The listing builds one solid part. Answer for the finished solid, in the listing's coordinates (mm). Face numbers are marked on the shaded views. A direction names the side the tool comes from. Round coordinates to 2 decimals unless told otherwise and drop trailing zeros. Loops run counter-clockwise (first coordinate to the right, second up) from the corner with the lowest first, then second, coordinate; pieces in that order, holes last. Notation, with made-up numbers: (55, 18) -> (84, 18) arc R28 cw to (84, 52) -> close; hole circle Ø3 at (41, 65.25). An arc over 180 degrees is marked (long way). Use a Markdown table: item, result. Add a question column.
Q1. Which of the six approach directions +Z, -Z, +X, -X, +Y, -Y give full straight-line access (tool end or side, diameter ignored) to the marked faces 1, 2 and 3?
Q2. Section A-A on x = -14.5 is taken. Give the vertices of the cut face in (y, z), then the cut area to 4 significant figures.
Q3. Given pin 1 Ø1.1 at (x, y) = (-13, 10.5) entering from +Z; pin 2 Ø14.5 at (x, y) = (-2, 2.5) entering from +Z; pin 3 Ø1.6 at (y, z) = (4, 1) entering from +X (3 decimals); pin 4 Ø1.1 at (y, z) = (5.5, 1) entering from -X (3 decimals), each flat-ended and moving along its own axis, determine where each tip first touches the part or whether it passes through.
Q4. Section B-B on x = 11.5 is taken. Give the vertices of the cut face in (y, z).
Q5. Consider line 1 (Y direction, x = 7, z = 0.6); line 2 (Y direction, x = 8.5, z = 2.85); line 3 (Y direction, x = 10, z = 0.5). Determine where each line is inside the solid, lowest interval first.
Q6. Section C-C on y = 5.5 is taken. Give the vertices of the cut face in (x, z) (3 decimals).
Q7. Section D-D on x = 0 is taken. Give the vertices of the cut face in (y, z).
from build123d import *

# Parameters (mm, degrees)
SKETCH_1_W            = 26.05
SKETCH_1_H            = 25
EXTRUDE_1_DEPTH       = 1.5
SKETCH_3_W            = 5.4
SKETCH_3_H            = 11.2
CUT_EXTRUDE_1_DEPTH   = 19.114928236
SKETCH_4_W            = 26.05
SKETCH_4_H            = 1.5
EXTRUDE_2_DEPTH       = 1.5
SKETCH_5_W            = 5.4
SKETCH_5_H            = 2
CUT_EXTRUDE_2_DEPTH   = 19.114928236
SKETCH_6_W            = 31
SKETCH_6_H            = 5.5
EXTRUDE_3_DEPTH       = 1.5
SKETCH_7_R            = 1
EXTRUDE_4_DEPTH       = 1.5
EXTRUDE_13_DEPTH      = 1
EXTRUDE_13_DEPTH_BACK = 1.5
SKETCH_10_W           = 4.95
SKETCH_10_H           = 6.5
FILLET_1_R            = 1
SKETCH_11_W           = 4.95
SKETCH_11_H           = 0.4
EXTRUDE_1_2_DEPTH     = 5
SKETCH_12_W           = 2.5
SKETCH_12_H           = 2.5
CUT_EXTRUDE_3_DEPTH   = 22.980744414
FILLET_2_R            = 3
FILLET_3_R            = 1
SKETCH_13_W           = 1
SKETCH_13_H           = 0.4
EXTRUDE_14_DEPTH      = 4
SKETCH_15_W           = 1.5
SKETCH_15_H           = 1
EXTRUDE_15_DEPTH      = 1
SKETCH_16_W           = 1
SKETCH_16_H           = 1
EXTRUDE_16_DEPTH      = 1.5
SKETCH_17_W           = 6.515
SKETCH_17_H           = 1
CUT_EXTRUDE_1_2_DEPTH = 1
SKETCH_18_W           = 0.5
SKETCH_18_H           = 1
EXTRUDE_17_DEPTH      = 2.17
SKETCH_20_W           = 0.5
SKETCH_20_H           = 1
EXTRUDE_18_DEPTH      = 2.17
SKETCH_21_W           = 6.515
SKETCH_21_H           = 1
SKETCH_21_H_2         = 1.095349757
CUT_EXTRUDE_4_DEPTH   = 1
SKETCH_22_W           = 0.5
SKETCH_22_H           = 1
EXTRUDE_19_DEPTH      = 2.17
SKETCH_23_W           = 0.5
SKETCH_23_H           = 1.095349757
EXTRUDE_20_DEPTH      = 2.17
FILLET_4_R            = 0.6


with BuildPart() as part:
    # Эскиз1 → Extrude 1 (new body)
    with BuildSketch(Plane.XY):
        Rectangle(SKETCH_1_W, SKETCH_1_H)
    extrude(amount=EXTRUDE_1_DEPTH)

    # Эскиз3 → Cut-Extrude 1 (cut, through all)
    with BuildSketch(Plane.XY.offset(1.5)):
        with Locations((10.325, 1.4)):
            Rectangle(SKETCH_3_W, SKETCH_3_H)
    extrude(amount=-CUT_EXTRUDE_1_DEPTH, mode=Mode.SUBTRACT)

    # Эскиз4 → Бобышка-Вытянуть2 (add)
    with BuildSketch(Plane.XY.offset(1.5)):
        with Locations((0, 11.75)):
            Rectangle(SKETCH_4_W, SKETCH_4_H)
    extrude(amount=EXTRUDE_2_DEPTH)

    # Эскиз5 → Вырез-Вытянуть2 (cut, through all)
    with BuildSketch(Plane.XY.offset(1.5)):
        with Locations((10.325, 10)):
            Rectangle(SKETCH_5_W, SKETCH_5_H)
    extrude(amount=-CUT_EXTRUDE_2_DEPTH, mode=Mode.SUBTRACT)

    # Эскиз6 → Бобышка-Вытянуть3 (add)
    with BuildSketch(Plane.XY.offset(1.5)):
        with Locations((-2.475, -9.75)):
            Rectangle(SKETCH_6_W, SKETCH_6_H)
    extrude(amount=EXTRUDE_3_DEPTH)

    # Эскиз7 → Бобышка-Вытянуть4 (add)
    with BuildSketch(Plane(origin=(13.025, 0, 0), x_dir=(0, 0, -1), z_dir=(1, 0, 0))):
        with Locations(Location((-1.132985358, -11.301432667, 0), (0, 0, 180))):
            Circle(SKETCH_7_R)
    extrude(amount=EXTRUDE_4_DEPTH)

    # Эскиз10 → Бобышка-Вытянуть13 (add, two sides: drawn at the far end of the back side and taken through both)
    with BuildSketch(Plane(origin=(0, 0, 1.5), x_dir=(-1, 0, 0), z_dir=(0, 0, -1)).offset(-EXTRUDE_13_DEPTH_BACK)):
        with Locations((15.5, -9.25)):
            Rectangle(SKETCH_10_W, SKETCH_10_H)
    extrude(amount=EXTRUDE_13_DEPTH + EXTRUDE_13_DEPTH_BACK)

    # Скругление1
    fillet_1_edges = [part.edges().sort_by_distance(p)[0] for p in [
        (-17.975, -12.5, 1.75),
        (-17.975, -6, 1.75),
        (-13.025, -6, 2.25),
    ]]
    fillet(fillet_1_edges, radius=FILLET_1_R - 0.0001)  # a hair under: the kernel refuses the full size

    # Эскиз11 → Extrude 1 2 (add)
    with BuildSketch(Plane(origin=(0, -6, 0), x_dir=(1, 0, 0), z_dir=(0, 1, 0))):
        with Locations((-15.5, -1.75)):
            Rectangle(SKETCH_11_W, SKETCH_11_H)
    extrude(amount=EXTRUDE_1_2_DEPTH)

    # Эскиз12 → Вырез-Вытянуть3 (cut, through all)
    with BuildSketch(Plane.XY.offset(1.95)):
        with Locations((-14.275, -4.75)):
            Rectangle(SKETCH_12_W, SKETCH_12_H)
    extrude(amount=-CUT_EXTRUDE_3_DEPTH, mode=Mode.SUBTRACT)

    # Скругление2
    fillet_2_edges = [part.edges().sort_by_distance(p)[0] for p in [
        (-17.975, -1, 1.75),
    ]]
    fillet(fillet_2_edges, radius=FILLET_2_R)

    # Скругление3
    fillet_3_edges = [part.edges().sort_by_distance(p)[0] for p in [
        (-13.025, -1, 1.75),
        (-13.025, -3.5, 1.75),
    ]]
    fillet(fillet_3_edges, radius=FILLET_3_R)

    # Эскиз13 → Бобышка-Вытянуть14 (add)
    with BuildSketch(Plane.XZ.offset(6)):
        with Locations((-17.475, 1.75)):
            Rectangle(SKETCH_13_W, SKETCH_13_H)
    extrude(amount=EXTRUDE_14_DEPTH)

    # Эскиз15 → Бобышка-Вытянуть15 (add)
    with BuildSketch(Plane.ZY.offset(13.025)):
        with Locations((0.75, 8.5)):
            Rectangle(SKETCH_15_W, SKETCH_15_H)
    extrude(amount=EXTRUDE_15_DEPTH)

    # Эскиз16 → Бобышка-Вытянуть16 (add)
    with BuildSketch(Plane.XY.offset(1.5)):
        with Locations((-13.525, 8.5)):
            Rectangle(SKETCH_16_W, SKETCH_16_H)
    extrude(amount=EXTRUDE_16_DEPTH)

    # Эскиз17 → Cut-Extrude 1 2 (cut)
    with BuildSketch(Plane.XY.offset(1.5)):
        with Locations((-9.7675, -2)):
            Rectangle(SKETCH_17_W, SKETCH_17_H)
        with Locations((4.3675, -2)):
            Rectangle(SKETCH_17_W, SKETCH_17_H)
        with Locations((-9.7675, 0.54)):
            Rectangle(SKETCH_17_W, SKETCH_17_H)
        with Locations((4.3675, 0.54)):
            Rectangle(SKETCH_17_W, SKETCH_17_H)
        with Locations((-9.7675, 3.08)):
            Rectangle(SKETCH_17_W, SKETCH_17_H)
        with Locations((4.3675, 3.08)):
            Rectangle(SKETCH_17_W, SKETCH_17_H)
        with Locations((-9.7675, 5.62)):
            Rectangle(SKETCH_17_W, SKETCH_17_H)
        with Locations((4.3675, 5.62)):
            Rectangle(SKETCH_17_W, SKETCH_17_H)
    extrude(amount=-CUT_EXTRUDE_1_2_DEPTH, mode=Mode.SUBTRACT)

    # Эскиз18 → Бобышка-Вытянуть17 (add)
    with BuildSketch(Plane(origin=(7.625, 0, 0), x_dir=(0, 0, -1), z_dir=(1, 0, 0))):
        with Locations((-0.25, 3.08)):
            Rectangle(SKETCH_18_W, SKETCH_18_H)
        with Locations((-0.25, 5.62)):
            Rectangle(SKETCH_18_W, SKETCH_18_H)
        with Locations((-0.25, 0.54)):
            Rectangle(SKETCH_18_W, SKETCH_18_H)
        with Locations((-0.25, -2)):
            Rectangle(SKETCH_18_W, SKETCH_18_H)
    extrude(amount=EXTRUDE_17_DEPTH)

    # Эскиз20 → Бобышка-Вытянуть18 (add)
    with BuildSketch(Plane.ZY.offset(13.025)):
        with Locations((0.25, 3.08)):
            Rectangle(SKETCH_20_W, SKETCH_20_H)
        with Locations((0.25, 5.62)):
            Rectangle(SKETCH_20_W, SKETCH_20_H)
        with Locations((0.25, 0.54)):
            Rectangle(SKETCH_20_W, SKETCH_20_H)
        with Locations((0.25, -2)):
            Rectangle(SKETCH_20_W, SKETCH_20_H)
    extrude(amount=EXTRUDE_18_DEPTH)

    # Эскиз21 → Вырез-Вытянуть4 (cut)
    with BuildSketch(Plane.XY.offset(1.5)):
        with Locations((-9.7675, 10.5)):
            Rectangle(SKETCH_21_W, SKETCH_21_H)
        with Locations((4.3675, 10.452325121)):
            Rectangle(SKETCH_21_W, SKETCH_21_H_2)
    extrude(amount=-CUT_EXTRUDE_4_DEPTH, mode=Mode.SUBTRACT)

    # Эскиз22 → Бобышка-Вытянуть19 (add)
    with BuildSketch(Plane.ZY.offset(13.025)):
        with Locations((0.25, 10.5)):
            Rectangle(SKETCH_22_W, SKETCH_22_H)
    extrude(amount=EXTRUDE_19_DEPTH)

    # Эскиз23 → Бобышка-Вытянуть20 (add)
    with BuildSketch(Plane(origin=(7.625, 0, 0), x_dir=(0, 0, -1), z_dir=(1, 0, 0))):
        with Locations((-0.25, 10.452325121)):
            Rectangle(SKETCH_23_W, SKETCH_23_H)
    extrude(amount=EXTRUDE_20_DEPTH)

    # Скругление4
    fillet_4_edges = [part.edges().sort_by_distance(p)[0] for p in [
        (-14.025, 8.5, 3),
    ]]
    fillet(fillet_4_edges, radius=FILLET_4_R)


solid = part.part
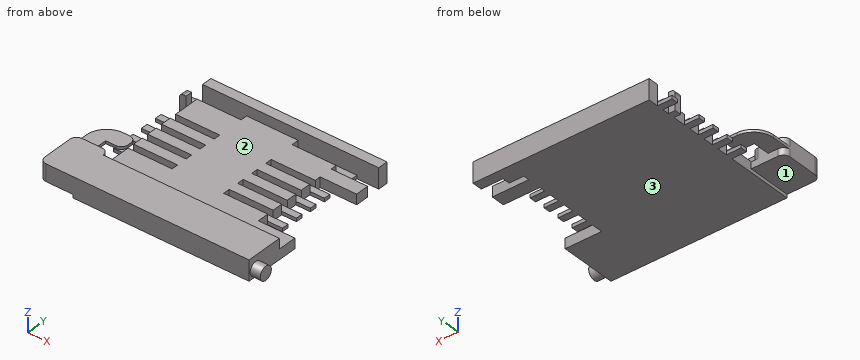
Checked values:
| question | item | result |
|---|---|---|
| 1 | face 1 | -Z, -X, -Y |
| 1 | face 2 | +Z, +X |
| 1 | face 3 | -Z, +X, -X, +Y, -Y |
| 2 | outline | (-12.5, 0.5) -> (-6, 0.5) -> (-6, 3) -> (-12.5, 3) -> close; (-3.5, 1.55) -> (-1, 1.55) -> (-1, 1.95) -> (-3.5, 1.95) -> close; (-2.5, 0) -> (-1.5, 0) -> (-1.5, 0.5) -> (-2.5, 0.5) -> close; (0.04, 0) -> (1.04, 0) -> (1.04, 0.5) -> (0.04, 0.5) -> close; (2.58, 0) -> (3.58, 0) -> (3.58, 0.5) -> (2.58, 0.5) -> close; (5.12, 0) -> (6.12, 0) -> (6.12, 0.5) -> (5.12, 0.5) -> close; (10, 0) -> (11, 0) -> (11, 0.5) -> (10, 0.5) -> close |
| 2 | area | 19.75 mm2 |
| 3 | pin 1 | stops at z = 3 |
| 3 | pin 2 | stops at z = 1.5 |
| 3 | pin 3 | stops at x = 9.795 |
| 3 | pin 4 | stops at x = -15.195 |
| 4 | outline | (-12.5, 0) -> (-4.2, 0) -> (-4.2, 1.5) -> (-7, 1.5) -> (-7, 3) -> (-12.5, 3) -> close; (7, 0) -> (9, 0) -> (9, 1.5) -> (7, 1.5) -> close; (11, 0) -> (12.5, 0) -> (12.5, 3) -> (11, 3) -> close |
| 5 | line 1 | y = -12.5 to -2.5, -1.5 to 0.04, 1.04 to 2.58, 3.58 to 5.12, 6.12 to 9.9, 11 to 12.5 |
| 5 | line 2 | y = -12.5 to -7, 11 to 12.5 |
| 5 | line 3 | y = -12.5 to -4.2, 7 to 9, 11 to 12.5 |
| 6 | outline | (-15.195, 0) -> (9.795, 0) -> (9.795, 0.5) -> (1.11, 0.5) -> (1.11, 1.5) -> (-6.51, 1.5) -> (-6.51, 0.5) -> (-15.195, 0.5) -> close |
| 7 | outline | (-12.5, 0) -> (12.5, 0) -> (12.5, 3) -> (11, 3) -> (11, 1.5) -> (-7, 1.5) -> (-7, 3) -> (-12.5, 3) -> close |
